Check sheet for the modelled part. Datum: model origin and axes. Units: mm. A direction names the side the tool comes from. Round coordinates to 2 decimals unless told otherwise and drop trailing zeros. Order: outer loops, then holes, each group sorted by start corner. A loop starts at its lowest first (then second) coordinate and runs counter-clockwise, first axis right, second up.
```python
from build123d import *

# Parameters (mm, degrees)
EXTRUDE_THIN1_DEPTH = 20
SKETCH2_R           = 2.5
CUT_EXTRUDE1_DEPTH  = 10
SKETCH3_R           = 1.5
CUT_EXTRUDE2_DEPTH  = 10


with BuildPart() as part:
    # Sketch1 → Extrude-Thin1 (new body)
    with BuildSketch(Plane(origin=(0, 0, 0), x_dir=(1, 0, 0), z_dir=(0, 1, 0))):
        Polygon((0, 0), (0, 12), (15, 12), (15, 10), (2, 10), (2, 0), align=None)
    extrude(amount=EXTRUDE_THIN1_DEPTH)

    # Sketch2 → Cut-Extrude1 (cut)
    with BuildSketch(Plane.ZY):
        with Locations((-5, 10)):
            Circle(SKETCH2_R)
    extrude(amount=-CUT_EXTRUDE1_DEPTH, mode=Mode.SUBTRACT)

    # Sketch3 → Cut-Extrude2 (cut)
    with BuildSketch(Plane(origin=(0, 0, -12), x_dir=(-1, 0, 0), z_dir=(0, 0, -1))):
        with Locations((-10, 17)):
            Circle(SKETCH3_R)
        with Locations((-10, 3)):
            Circle(SKETCH3_R)
    extrude(amount=-CUT_EXTRUDE2_DEPTH, mode=Mode.SUBTRACT)


solid = part.part
```
Item 1: Sectioned sample at B-B (y = 3). Record the cut outline in (x, z).
Answer:
outline: (0, -12) - (8.5, -12) - (8.5, -10) - (2, -10) - (2, 0) - (0, 0) - close; (11.5, -12) - (15, -12) - (15, -10) - (11.5, -10) - close
Item 2: Sectioned sample at D-D (x = 10). Record the cut outline in (y, z).
Answer:
outline: (0, -12) - (1.5, -12) - (1.5, -10) - (0, -10) - close; (4.5, -12) - (15.5, -12) - (15.5, -10) - (4.5, -10) - close; (18.5, -12) - (20, -12) - (20, -10) - (18.5, -10) - close
Item 3: Go/stop test with flat-tipped pins: P1, Ø5, axis at x = 7, y = 5, coming from the +Z side; P2, Ø4.5, axis at y = 10, z = -5, coming from the -X side; P3, Ø3, axis at y = 14, z = -5.5, coming from the +X side. Record where each tip stops, or that it passes through.
Answer:
P1: stops at z = -10
P2: passes through
P3: stops at x = 2
Item 4: Release check for a two-part mould opening along Y. For faces 3 (the flat face through (5, 0, -11)), 4 (the cylindrical face through (0.99, 7.78, -3.85)), 5 (the flat face through (5, 20, -11)), 6 (the flat face through (9, 10, -10)) record: released by +Y, released by -Y, zero draft, split by the parting line, or undercut.
Answer:
face 3: released by -Y
face 4: undercut
face 5: released by +Y
face 6: zero draft
Item 5: Scan lines: line 1 along Y through (x, z) = (10, -11.35); line 2 along Y through (x, z) = (1.25, -5); line 3 along X through (y, z) = (9.5, -0.75). Record each from-to range of solid material in increasing order.
Answer:
line 1: y = 0 to 1.5, 4.5 to 15.5, 18.5 to 20
line 2: y = 0 to 7.5, 12.5 to 20
line 3: x = 0 to 2
Item 6: Access from +Z, -Z, +X, -X, +Y, -Y to the whole of each face (thin tool, end or side, straight path). Record for faces 1 (the flat face through (7, 10, -12)), 2 (the flat face through (2, 7.6, -6.2)).
Answer:
face 1: -Z, +X, -X, +Y, -Y
face 2: +Z, +X, +Y, -Y
Item 7: Sectioned sample at C-C (x = 1.5). Record the cut outline in (y, z), and give its area (3 significant figures).
Answer:
outline: (0, -12) - (20, -12) - (20, 0) - (0, 0) - close; hole circle Ø5 at (10, -5)
area: 220 mm2
Item 8: Sectioned sample at A-A (z = -5). Record the cut outline in (x, y), and give its area (3 significant figures).
Answer:
outline: (0, 0) - (2, 0) - (2, 7.5) - (0, 7.5) - close; (0, 12.5) - (2, 12.5) - (2, 20) - (0, 20) - close
area: 30.0 mm2
